Read the model definition and answer for the solid it produces. Units are mm, in the model's axes. A direction names the side the tool comes from. Give positions to 0.01 mm unless a question says otherwise; leave off trailing zeros. Write each loop counter-clockwise with the first axis right and the second up, starting at its lowest first coordinate (ties: lowest second). Pieces come first, ordered by that corner, then holes. Notation, with made-up numbers: (-14, 36) -> (1, 36) arc R22 ccw to (1, 42) -> close; hole circle Ø5 at (8, 4). An arc over 180 degrees is marked (long way). Put each result on its own line as item: value. Start each with the question number.
Autodesk Inventor part; units mm, degrees
ref_plane "YZ Plane" through (0, 0, 0) normal (1, 0, 0) x (0, 1, 0)
ref_plane "XZ Plane" through (0, 0, 0) normal (0, 1, 0) x (-1, 0, 0)
ref_plane "XY Plane" through (0, 0, 0) normal (0, 0, 1) x (1, 0, 0)
sketch "Sketch1" plane through (0, 0, 0) normal (0, 0, 1) x (1, 0, 0)
  line L0 (0, 0) -> (58, 0)
  line L1 (58, 0) -> (58, 98)
  line L2 (58, 98) -> (0, 98)
  line L3 (0, 98) -> (0, 0)
  line L4 (15, 62) -> (43, 62)
  line L5 (43, 62) -> (43, 12)
  line L6 (43, 12) -> (15, 12)
  line L7 (15, 12) -> (15, 62)
  circle A0 centre (9, 37) radius 2.5
  circle A1 centre (49, 37) radius 2.5
  line L8 (9, 37) -> (49, 37) construction
  line L9 (3, 86) -> (27, 86)
  line L10 (27, 86) -> (27, 74)
  line L11 (27, 74) -> (3, 74)
  line L12 (3, 74) -> (3, 86)
  circle A2 centre (-8.5, 49) radius 2.5
  circle A3 centre (66.5, 49) radius 2.5
  line L13 (-8.5, 49) -> (66.5, 49) construction
  circle A4 centre (-8.5, 49) radius 5 construction
  circle A5 centre (66.5, 49) radius 5 construction
  line L14 (0, 0) -> (-13.3155, 47.6544)
  line L15 (0, 98) -> (-13.3155, 50.3456)
  line L16 (58, 98) -> (71.3155, 50.3456)
  line L17 (58, 0) -> (71.3155, 47.6544)
  arc A6 (-13.3155, 50.3456) -> (-13.3155, 47.6544) centre (-8.5, 49) ccw
  arc A7 (71.3155, 47.6544) -> (71.3155, 50.3456) centre (66.5, 49) ccw
  line L18 (32, 90.5) -> (55, 90.5)
  line L19 (55, 90.5) -> (55, 69.5)
  line L20 (55, 69.5) -> (32, 69.5)
  line L21 (32, 69.5) -> (32, 90.5)
  line L22 (3, 80) -> (55, 80) construction
  point P0 (29, 62)
  point P1 (29, 98)
  point P2 (29, 37)
  point P3 (15, 37)
  point P4 (29, 49)
  point P5 (0, 49)
  point P6 (29, 80)
  dimension "d0" = 58
  dimension "d1" = 98
  dimension "d2" = 28
  dimension "d3" = 50
  dimension "d4" = 12
  dimension "d5" = 5
  dimension "d6" = 5
  dimension "d7" = 40
  dimension "d9" = 24
  dimension "d10" = 12
  dimension "d12" = 12
  dimension "d13" = 5
  dimension "d14" = 5
  dimension "d15" = 75
  dimension "d16" = 10
  dimension "d17" = 10
  dimension "d18" = 23
  dimension "d19" = 21
  dimension "d20" = 5
extrude "Extrusion1" add sketch "Sketch1" against normal blind 3
extrude "Extrusion2" add sketch "Sketch1" along normal blind 25 contours L3 L2 L1 L0
fillet "Fillet1" radius 5 4 edges at (58, 98, 12.5) (58, 0, 12.5) (0, 0, 12.5) (0, 98, 12.5)
sketch "Sketch2" plane through (0, 0, 0) normal (0, 0, 1) x (1, 0, 0)
  circle A0 centre (49, 37) radius 2.5
  circle A1 centre (9, 37) radius 2.5
  line L0 (0, 5) -> (0, 93)
  line L1 (0, 32.5) -> (13.5, 32.5)
  line L2 (13.5, 32.5) -> (13.5, 41.5)
  line L3 (13.5, 41.5) -> (0, 41.5)
  line L4 (0, 41.5) -> (0, 32.5)
  line L5 (58, 5) -> (58, 93)
  line L6 (58, 32.5) -> (44.5, 32.5)
  line L7 (44.5, 32.5) -> (44.5, 41.5)
  line L8 (44.5, 41.5) -> (58, 41.5)
  line L9 (58, 41.5) -> (58, 32.5)
  line L10 (15, 62) -> (15, 12)
  line L11 (43, 12) -> (43, 62)
  point P0 (0, 0)
  point P1 (13.5, 37)
  point P2 (44.5, 37)
  dimension "d29" = 4.5
  dimension "d30" = 4.5
  dimension "d31" = 9
extrude "Extrusion3" cut sketch "Sketch2" along normal through all
sketch "Sketch3" plane through (0, 0, -3) normal (0, 0, -1) x (-1, 0, 0)
  circle A0 centre (-29, -5) radius 2.5 construction
  circle A1 centre (-29, 103) radius 2.5 construction
  line L0 (0, 98) -> (-58, 98)
  line L1 (-58, 0) -> (0, 0)
  line L2 (-58, 98) -> (-29.6325, 105.4187)
  line L3 (0, 98) -> (-28.3675, 105.4187)
  line L4 (0, 0) -> (-28.3675, -7.4187)
  line L5 (-58, 0) -> (-29.6325, -7.4187)
  arc A2 (-29.6325, -7.4187) -> (-28.3675, -7.4187) centre (-29, -5) ccw
  arc A3 (-28.3675, 105.4187) -> (-29.6325, 105.4187) centre (-29, 103) ccw
  point P0 (-29, 98)
  dimension "d34" = 5
  dimension "d35" = 5
  dimension "d36" = 5
  dimension "d37" = 5
extrude "Extrusion4" add sketch "Sketch3" against normal blind 3
fillet "Fillet2" radius 5 4 edges at (0, 98, -1.5) (58, 98, -1.5) (58, 0, -1.5) (0, 0, -1.5)
sketch "Sketch4" plane through (0, 0, -3) normal (0, 0, -1) x (-1, 0, 0)
  line L0 (-15, 62) -> (-15, 12)
  line L1 (-15, 12) -> (-43, 12)
  line L2 (-43, 12) -> (-43, 62)
  line L3 (-43, 62) -> (-15, 62)
  line L4 (-32, 90.5) -> (-32, 69.5)
  line L5 (-32, 69.5) -> (-55, 69.5)
  line L6 (-55, 69.5) -> (-55, 90.5)
  line L7 (-55, 90.5) -> (-32, 90.5)
  line L8 (-3, 86) -> (-3, 74)
  line L9 (-3, 74) -> (-27, 74)
  line L10 (-27, 74) -> (-27, 86)
  line L11 (-27, 86) -> (-3, 86)
  circle A0 centre (-49, 37) radius 2.5
  circle A1 centre (-9, 37) radius 2.5
  circle A2 centre (-66.5, 49) radius 2.5
  circle A3 centre (8.5, 49) radius 2.5
  arc A4 (-2.7778, -0.7265) -> (0.7727, 2.7653) centre (-4.0429, 4.1109) ccw
  line L12 (0.7727, 2.7653) -> (13.3155, 47.6544)
  arc A5 (13.3155, 47.6544) -> (13.3155, 50.3456) centre (8.5, 49) ccw
  line L13 (13.3155, 50.3456) -> (0.7727, 95.2347)
  arc A6 (0.7727, 95.2347) -> (-2.7778, 98.7265) centre (-4.0429, 93.8891) ccw
  line L14 (-28.3675, 105.4187) -> (-2.7778, 98.7265)
  arc A7 (-28.3675, 105.4187) -> (-29.6325, 105.4187) centre (-29, 103) ccw
  line L15 (-55.2222, 98.7265) -> (-29.6325, 105.4187)
  arc A8 (-55.2222, 98.7265) -> (-58.7727, 95.2347) centre (-53.9571, 93.8891) ccw
  line L16 (-58.7727, 95.2347) -> (-71.3155, 50.3456)
  arc A9 (-71.3155, 50.3456) -> (-71.3155, 47.6544) centre (-66.5, 49) ccw
  line L17 (-71.3155, 47.6544) -> (-58.7727, 2.7653)
  arc A10 (-58.7727, 2.7653) -> (-55.2222, -0.7265) centre (-53.9571, 4.1109) ccw
  line L18 (-55.2222, -0.7265) -> (-29.6325, -7.4187)
  arc A11 (-29.6325, -7.4187) -> (-28.3675, -7.4187) centre (-29, -5) ccw
  line L19 (-28.3675, -7.4187) -> (-2.7778, -0.7265)
  arc A12 (-27.3554, 109.2885) -> (-30.6446, 109.2885) centre (-29, 103) ccw
  line L20 (-27.3554, 109.2885) -> (-1.7658, 102.5963)
  arc A13 (4.6251, 96.3111) -> (-1.7658, 102.5963) centre (-4.0429, 93.8891) ccw
  line L21 (4.6251, 96.3111) -> (17.168, 51.422)
  arc A14 (17.168, 46.578) -> (17.168, 51.422) centre (8.5, 49) ccw
  line L22 (17.168, 46.578) -> (4.6251, 1.6889)
  arc A15 (-1.7658, -4.5963) -> (4.6251, 1.6889) centre (-4.0429, 4.1109) ccw
  line L23 (-1.7658, -4.5963) -> (-27.3554, -11.2885)
  arc A16 (-30.6446, -11.2885) -> (-27.3554, -11.2885) centre (-29, -5) ccw
  line L24 (-30.6446, -11.2885) -> (-56.2342, -4.5963)
  arc A17 (-62.6251, 1.6889) -> (-56.2342, -4.5963) centre (-53.9571, 4.1109) ccw
  line L25 (-62.6251, 1.6889) -> (-75.168, 46.578)
  arc A18 (-75.168, 51.422) -> (-75.168, 46.578) centre (-66.5, 49) ccw
  line L26 (-75.168, 51.422) -> (-62.6251, 96.3111)
  arc A19 (-56.2342, 102.5963) -> (-62.6251, 96.3111) centre (-53.9571, 93.8891) ccw
  line L27 (-56.2342, 102.5963) -> (-30.6446, 109.2885)
  point P0 (0, 0)
  dimension "d41" = 4
extrude "Extrusion5" add sketch "Sketch4" against normal blind 3 contours L20 A13 L21 A14 L22 A15 L23 A16 L24 A17 L25 A18 L26 A19 L27 A12
sketch "Sketch6" plane through (0, 0, -3) normal (0, 0, -1) x (-1, 0, 0)
  line L0 (-29, 118.6904) -> (17.5, 91.8437) construction
  line L1 (17.5, 91.8437) -> (17.5, 38.1501) construction
  line L2 (17.5, 38.1501) -> (-29, 11.3033) construction
  line L3 (-29, 11.3033) -> (-75.5, 38.1501) construction
  line L4 (-75.5, 38.1501) -> (-75.5, 91.8437) construction
  line L5 (-75.5, 91.8437) -> (-29, 118.6904) construction
  line L6 (-29, -20.6904) -> (-75.5, 6.1563) construction
  line L7 (-75.5, 6.1563) -> (-75.5, 59.8499) construction
  line L8 (-75.5, 59.8499) -> (-29, 86.6967) construction
  line L9 (-29, 86.6967) -> (17.5, 59.8499) construction
  line L10 (17.5, 59.8499) -> (17.5, 6.1563) construction
  line L11 (17.5, 6.1563) -> (-29, -20.6904) construction
  line L12 (-15, 12) -> (-43, 12) construction
  arc A0 (-75.168, 51.422) -> (-75.168, 46.578) centre (-66.5, 49) ccw construction
  line L13 (-75.5, 59.8499) -> (-75.5, 38.1501) construction
  line L14 (17.5, 59.8499) -> (17.5, 38.1501) construction
  arc A1 (17.168, 46.578) -> (17.168, 51.422) centre (8.5, 49) ccw construction
  arc A2 (4.6251, 96.3111) -> (-1.7658, 102.5963) centre (-4.0429, 93.8891) ccw construction
  arc A3 (-1.7658, -4.5963) -> (4.6251, 1.6889) centre (-4.0429, 4.1109) ccw construction
  line L15 (-72.6977, 49) -> (-55.2357, 96.3111)
  line L16 (-55.2357, 96.3111) -> (0, 98)
  line L17 (0, 98) -> (14.2585, 49.0151)
  line L18 (14.2585, 49.0151) -> (2.9964, 0)
  line L19 (2.9964, 0) -> (-59.2966, 2.9606)
  line L20 (-59.2966, 2.9606) -> (-72.6977, 49)
  line L21 (-75.5, 91.8437) -> (-75.5, 6.1563)
  line L22 (-75.5, 6.1563) -> (-29, -20.6904)
  line L23 (-29, -20.6904) -> (17.5, 6.1563)
  line L24 (17.5, 91.8437) -> (17.5, 6.1563)
  line L25 (17.5, 91.8437) -> (-29, 118.6904)
  line L26 (-29, 118.6904) -> (-75.5, 91.8437)
  point P0 (0, 0)
  point P1 (-29, 64.9969)
  point P2 (-29, 33.0031)
  point P3 (-29, 12)
extrude "Extrusion7" add sketch "Sketch6" against normal blind 3
sketch "Sketch7" plane through (0, 0, -3) normal (0, 0, -1) x (-1, 0, 0)
  line L0 (-75.5, 91.8437) -> (-29, 118.6904)
  circle A0 centre (-29, 118.6904) radius 10
  point P0 (0, 0)
  dimension "d48" = 20
extrude "Extrusion8" cut sketch "Sketch7" against normal through all
sketch "Sketch9" plane through (0, 0, 25) normal (0, 0, 1) x (1, 0, 0)
  line L0 (26.5, 12) -> (26.5, -20.6904)
  line L1 (26.5, -20.6904) -> (31.5, -20.6904)
  line L2 (31.5, -20.6904) -> (31.5, 12)
  line L3 (31.5, 12) -> (26.5, 12)
  line L4 (29, 12) -> (29, -20.6904) construction
  line L5 (43, 12) -> (15, 12)
  point P0 (0, 0)
  dimension "d51" = 5
extrude "Extrusion9" cut sketch "Sketch9" against normal through all
sketch "Sketch11" plane through (0, 0, 0) normal (0, 0, 1) x (1, 0, 0)
  line L0 (31.5, 0) -> (31.5, -19.2471)
  line L1 (31.5, 0) -> (53, 0)
  line L2 (31.5, -19.2471) -> (75.5, 6.1563)
  line L3 (31.5, 0) -> (53, 0)
  line L4 (36.5, 0) -> (36.5, -16.3603)
  line L5 (31.5, -19.2471) -> (36.5, -16.3603)
  line L6 (31.5, 0) -> (36.5, 0)
  point P0 (0, 0)
  dimension "d54" = 5
extrude "Extrusion10" add sketch "Sketch11" along normal blind 5
sketch "Sketch12" plane through (0, 0, 5) normal (0, 0, 1) x (1, 0, 0)
  line L0 (31.5, -19.2471) -> (75.5, 6.1563)
  line L1 (31.5, -19.2471) -> (29, -20.6904)
  line L2 (29, -20.6904) -> (26.5, -19.2471)
  line L3 (-17.5, 6.1563) -> (26.5, -19.2471)
  line L4 (-17.5, 6.1563) -> (26.5, -19.2471)
  line L5 (21.5, -16.3603) -> (21.5, 0)
  line L6 (5, 0) -> (26.5, 0)
  line L7 (21.5, 0) -> (36.5, 0)
  line L8 (36.5, 0) -> (36.5, -16.3603)
  line L9 (31.5, 0) -> (31.5, -19.2471)
  line L10 (31.5, -19.2471) -> (36.5, -16.3603)
  line L11 (36.5, -16.3603) -> (36.5, 0)
  line L12 (31.5, 0) -> (36.5, 0)
  line L13 (26.5, -19.2471) -> (26.5, 0)
  line L14 (21.5, -16.3603) -> (26.5, -19.2471)
  line L15 (29, -20.6904) -> (36.5, -16.3603)
  line L16 (21.5, 0) -> (36.5, 0)
  line L17 (31.5, 0) -> (53, 0)
  line L18 (21.5, -16.3603) -> (29, -20.6904)
  line L19 (29, -20.6904) -> (36.5, -16.3603)
  line L20 (36.5, -16.3603) -> (36.5, 0)
  line L21 (21.5, 0) -> (21.5, -16.3603)
  point P0 (0, 0)
  dimension "d57" = 5
extrude "Extrusion11" add sketch "Sketch12" along normal blind 5
sketch "Sketch13" plane through (5, 0, 0) normal (0, -1, 0) x (1, 0, 0)
  line L0 (21.5, 25) -> (21.5, -3)
  line L1 (0, 0) -> (21.5, 0)
  line L2 (21.5, 25) -> (11.5, 25)
  line L3 (11.5, 25) -> (11.5, 0)
  line L4 (11.5, 0) -> (21.5, 0)
  line L5 (21.5, 0) -> (21.5, 25)
  point P0 (-5, 0)
  dimension "d60" = 10
extrude "Extrusion12" cut sketch "Sketch13" against normal blind 15
sketch "Sketch14" plane through (21.5, 0, 5) normal (0, 1, 0) x (1, 0, 0)
  line L0 (10, -5) -> (10, 0)
  line L1 (10, 0) -> (0, 0)
  line L2 (0, 0) -> (0, -5)
  line L3 (0, -5) -> (10, -5)
  point P0 (-21.5, 5)
extrude "Extrusion13" add sketch "Sketch14" along normal blind 12
sketch "Sketch15" plane through (0, 0, 0) normal (0, 0, 1) x (1, 0, 0)
  line L0 (36.5, 0) -> (53, 0)
  line L1 (36.5, 0) -> (21.5, 0)
  line L2 (21.5, 0) -> (21.5, -20.6904)
  line L3 (21.5, -20.6904) -> (36.5, -20.6904)
  line L4 (36.5, -20.6904) -> (36.5, 0)
  point P0 (0, 0)
  point P1 (21.5, -16.3603)
  point P2 (29, -20.6904)
  point P3 (29, -20.6904)
extrude "Extrusion14" cut sketch "Sketch15" along normal through all
chamfer "Chamfer1" distance 2 angle 45 1 edges at (21.5, 6, 5)
properties part number "BA27" material "ABS Plastic"
1) A cutting plane is placed at B-B on z = 21.25. State how many separate pieces and enclosed holes the cut face has, and give its area (3 significant figures).
2) A cutting plane is placed at D-D on x = 9. Give the vertices of the cut face in (y, z), and give its area (3 significant figures).
3) A cutting plane is placed at C-C on y = 49. Give the vertices of the cut face in (x, z).
4) A cutting plane is placed at A-A on y = 78. Give the vertices of the cut face in (x, z), and give its area (3 significant figures).
5) For a pull along Y with two mould halves and no side action, classify faces 1 (the face through (9, 50, 25)), 2 (the face through (44.5, 37, 12)), 3 (the face through (4.808, -6.723, -1.521)) as pulls with the +Y half, pulls with the -Y half, needs draft (parallel to the pull), parting line crosses it, or undercut.
6) Each of these flat-tipped pins is pushed along its axis until it touches: pin 1 Ø12.5 at (y, z) = (70.5, 14.5) entering from -X; pin 2 Ø12 at (x, y) = (58, 98) entering from +Z; pin 3 Ø3 at (y, z) = (37, 17.5) entering from +X; pin 4 Ø3 at (y, z) = (1.5, 11) entering from +X. Where does it stop, or does it pass through?
7) For faces 4 (the face through (51, 41.5, 12)), 5 (the face through (15, 74, 11)), 6 (the face through (26.5, -3, -1)), 7 (the face through (29, 98, 12)), 8 (the face through (56, 1, 13)), determine the directions among +Z, -Z, +X, -X, +Y, -Y from which every point of the face is accessible in a straight line to the end or side of a thin tool.
8) Straight lines are drawn through the part: line 1 (Y direction, x = 17.5, z = 20.5); line 2 (X direction, y = 88.5, z = 22.75); line 3 (Y direction, x = 41.5, z = 18). For each, find the intervals that lie inside material, in ascending order. Write a range as [from, to].
Results found:
1. separate pieces: 1
1. enclosed holes: 2
1. area: 3,070 mm²
2. outline: (-9.14, -3) -> (34.5, -3) -> (34.5, 0) -> (32.5, 0) -> (32.5, 25) -> (0, 25) -> (0, 0) -> (-9.14, 0) -> close; (39.5, -3) -> (74, -3) -> (74, 25) -> (41.5, 25) -> (41.5, 0) -> (39.5, 0) -> close; (86, -3) -> (107.14, -3) -> (107.14, 0) -> (98, 0) -> (98, 25) -> (86, 25) -> close
2. area: 2,220 mm²
3. outline: (-17.5, -3) -> (-11, -3) -> (-11, 0) -> (-17.5, 0) -> close; (-6, -3) -> (15, -3) -> (15, 25) -> (0, 25) -> (0, 0) -> (-6, 0) -> close; (43, -3) -> (64, -3) -> (64, 0) -> (58, 0) -> (58, 25) -> (43, 25) -> close; (69, -3) -> (75.5, -3) -> (75.5, 0) -> (69, 0) -> close
4. outline: (-17.5, -3) -> (3, -3) -> (3, 25) -> (0, 25) -> (0, 0) -> (-17.5, 0) -> close; (27, -3) -> (32, -3) -> (32, 25) -> (27, 25) -> close; (55, -3) -> (75.5, -3) -> (75.5, 0) -> (58, 0) -> (58, 25) -> (55, 25) -> close
4. area: 413 mm²
5. face 1: needs draft
5. face 2: undercut
5. face 3: pulls with the -Y half
6. pin 1: stops at x = 0
6. pin 2: stops at z = 25
6. pin 3: stops at x = 44.5
6. pin 4: stops at x = 57.58
7. face 4: +Z, +X
7. face 5: +Z, -Z
7. face 6: -Z, -Y
7. face 7: +Z, +X, -X, +Y
7. face 8: +Z, +X, -Y
8. line 1: y = [62, 74], [86, 98]
8. line 2: x = [0, 32], [55, 58]
8. line 3: y = [0, 12], [62, 69.5], [90.5, 98]
